The drawing under review shows one solid part. Ordinate dimensions are in mm from its lowest x, y, z. A direction names the side the tool comes from. Give positions to 0.01 mm unless a question says otherwise; leave off trailing zeros. Loops run counter-clockwise (first coordinate to the right, second up) from the corner with the lowest first, then second, coordinate; pieces in that order, holes last. Notation, with made-up numbers: (31, 22) - (44, 22) arc R11 cw to (44, 36) - close; hole circle Ø3 at (-15.75, 11). An arc over 180 degrees is marked (long way). Return JSON: item names as keys, results as strings. Group by question number.
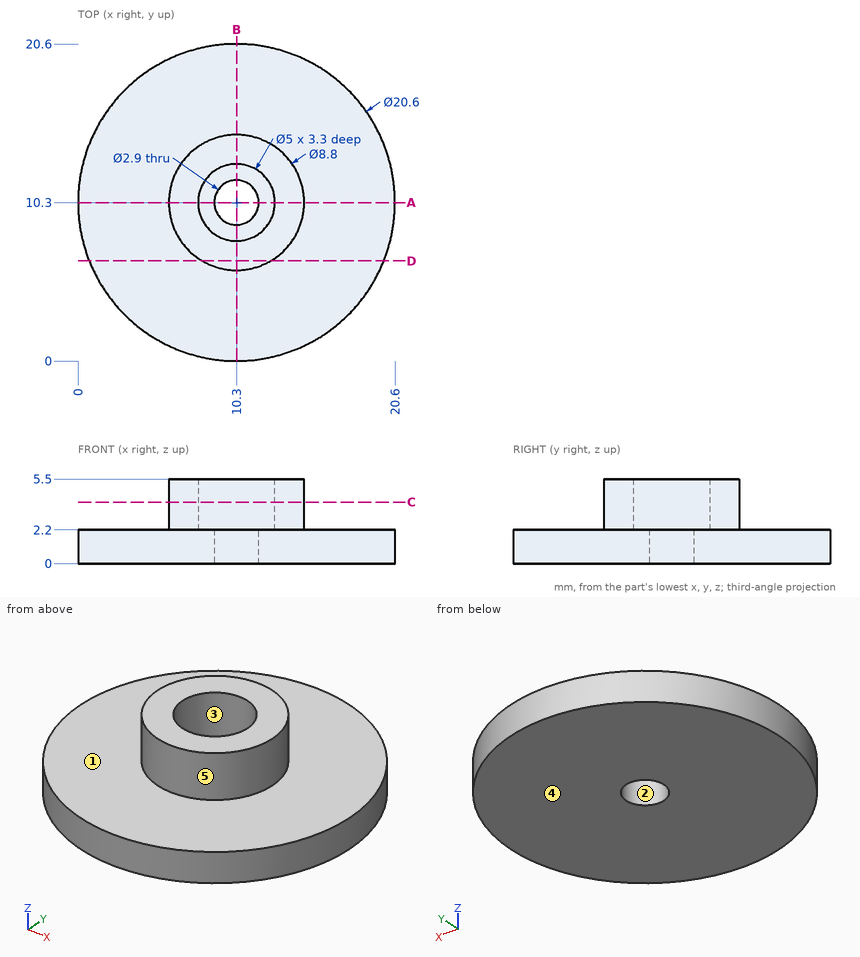
1) We need section D-D, the plane y = 6.5. Write out the cut boundary in (x, z), plus the area to 3 significant figures.
2) Draft analysis for pull direction Y (two halves, no side actions). For the marked faces 3, 4 and 5, state which applies: +Y half, -Y half, draft (parallel to the pull), parting line (faces both ways), or undercut.
3) Tool access review of the marked faces 1 and 2: name each direction out of +Z, -Z, +X, -X, +Y, -Y from which nothing blocks a thin tool from reaching the whole face with its end or side.
4) We need section C-C, the plane z = 4. Write out the cut boundary in (x, y), plus the area to 3 significant figures.
5) To check wall thickness, follow line 1 (Y direction, x = 10.3, z = 1.7); line 2 (Z direction, x = 7, y = 5.75); line 3 (Y direction, x = 10.3, z = 4.15). State the ranges of each line that lie inside material, in increasing order.
6) For pin 1 Ø2 at (x, z) = (14.5, 3.5) entering from +Y; pin 2 Ø1.5 at (x, z) = (11.5, 0.5) entering from +Y; pin 3 Ø3 at (y, z) = (2.5, 5) entering from +X; pin 4 Ø1.5 at (y, z) = (17.5, 1) entering from +X, all flat-tipped, find the tip position at first contact; note any pin that passes through.
7) We need section A-A, the plane y = 10.3. Write out the cut boundary in (x, z).
Findings:
{
 "1": {"outline": "(0.73, 0) - (19.87, 0) - (19.87, 2.2) - (12.52, 2.2) - (12.52, 5.5) - (8.08, 5.5) - (8.08, 2.2) - (0.73, 2.2) - close", "area": "56.8 mm^2"},
 "2": {"face 3": "undercut", "face 4": "draft", "face 5": "parting line"},
 "3": {"face 1": "+Z", "face 2": "+Z, -Z"},
 "4": {"outline": "circle Ø8.8 at (10.3, 10.3); hole circle Ø5 at (10.3, 10.3)", "area": "41.2 mm^2"},
 "5": {"line 1": "y = 0 to 8.85, 11.75 to 20.6", "line 2": "z = 0 to 2.2", "line 3": "y = 5.9 to 7.8, 12.8 to 14.7"},
 "6": {"pin 1": "stops at y = 13.32", "pin 2": "stops at y = 20.59", "pin 3": "passes through", "pin 4": "stops at x = 18.33"},
 "7": {"outline": "(0, 0) - (8.85, 0) - (8.85, 2.2) - (7.8, 2.2) - (7.8, 5.5) - (5.9, 5.5) - (5.9, 2.2) - (0, 2.2) - close; (11.75, 0) - (20.6, 0) - (20.6, 2.2) - (14.7, 2.2) - (14.7, 5.5) - (12.8, 5.5) - (12.8, 2.2) - (11.75, 2.2) - close"}
}
